Check sheet for the drawn part. Datum: minimum x, y, z corner. Units: mm. Round coordinates to 2 decimals unless told otherwise and drop trailing zeros. Order: outer loops, then holes, each group sorted by start corner. A loop starts at its lowest first (then second) coordinate and runs counter-clockwise, first axis right, second up. Notation, with made-up numbers: (20, 63) -> (33, 63) arc R21 cw to (33, 67) -> close; hole circle Ø2 at (6, 7.5). An arc over 180 degrees is marked (long way). Use CSV: the item, a comma, the result in double quotes.
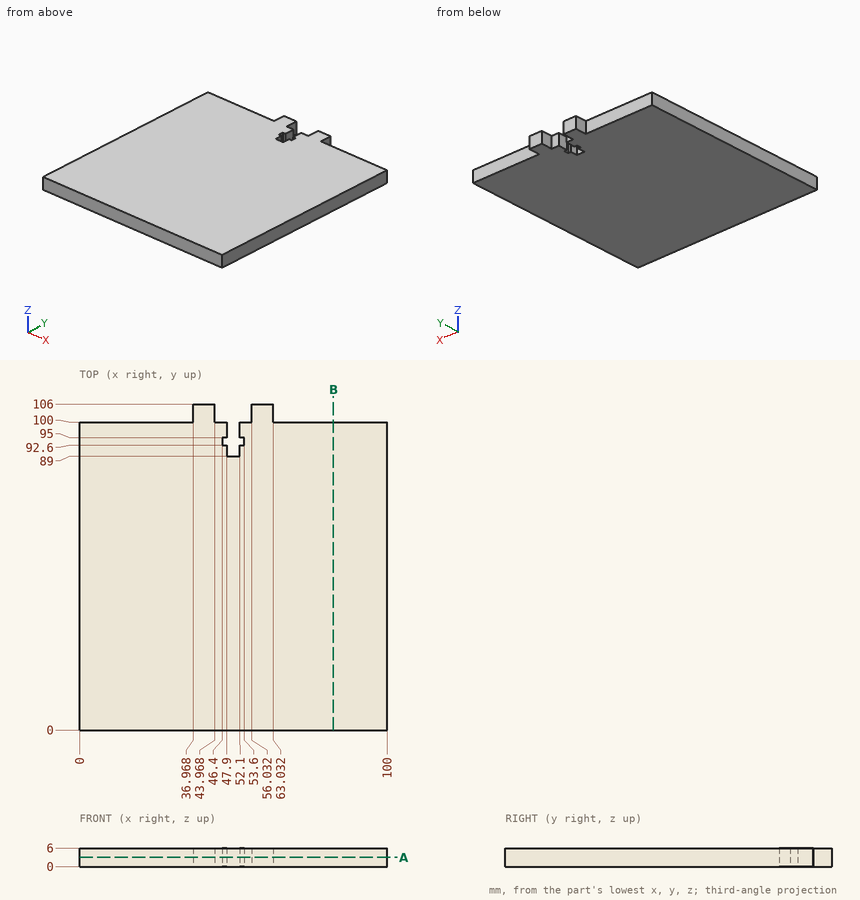
Q1. Go/stop test with flat-tipped pins: pin 1 (2 mm diameter, centred on x = 67.5, z = 2, fed in from +Y); pin 2 (3 mm diameter, centred on y = 102, z = 3, fed in from +X). Record where each tip stops, or that it passes through.
Result sheet:
pin 1,"stops at y = 100"
pin 2,"stops at x = 63.03"
Q2. Scan lines: L1, parallel to Y at x = 17, z = 4.4; L2, parallel to X at y = 93, z = 4.6. Record each from-to range of solid material in increasing order.
Result sheet:
L1,"y = 0 to 100"
L2,"x = 0 to 46.4, 53.6 to 100"
Q3. Sectioned sample at A-A, the plane z = 3. Enter the section's corners in (x, y).
Result sheet:
outline,"(0, 0) -> (100, 0) -> (100, 100) -> (63.03, 100) -> (63.03, 106) -> (56.03, 106) -> (56.03, 100) -> (52.1, 100) -> (52.1, 95) -> (53.6, 95) -> (53.6, 92.6) -> (52.1, 92.6) -> (52.1, 89) -> (47.9, 89) -> (47.9, 92.6) -> (46.4, 92.6) -> (46.4, 95) -> (47.9, 95) -> (47.9, 100) -> (43.97, 100) -> (43.97, 106) -> (36.97, 106) -> (36.97, 100) -> (0, 100) -> close"
Q4. Sectioned sample at B-B, the plane x = 82.5. Enter the section's corners in (y, z), then the cut area to 3 significant figures.
Result sheet:
outline,"(0, 0) -> (100, 0) -> (100, 6) -> (0, 6) -> close"
area,"600 mm^2"
